Autodesk Inventor part; units mm, degrees
ref_plane "YZ Plane" through (0, 0, 0) normal (1, 0, 0) x (0, 1, 0)
ref_plane "XZ Plane" through (0, 0, 0) normal (0, 1, 0) x (-1, 0, 0)
ref_plane "XY Plane" through (0, 0, 0) normal (0, 0, 1) x (1, 0, 0)
sketch "Sketch1" plane through (0, 0, 0) normal (0, 0, 1) x (1, 0, 0)
  circle A0 centre (0, 0) radius 83.5
  circle A1 centre (0, 0) radius 140
  dimension "d22" = 167
  dimension "d23" = 280
extrude "Plate1" add sketch "Sketch1" along normal blind 4
sketch "Sketch5" plane through (0, 0, 4) normal (0, 0, 1) x (1, 0, 0)
  circle A0 centre (84.8528, 84.8528) radius 9
  circle A1 centre (0, 0) radius 120 construction
  line L0 (84.8528, 84.8528) -> (0, 0) construction
  line L1 (0, 0) -> (0, 120) construction
  dimension "d24" = 18
  dimension "d25" = 240
  dimension "d31" = 45
extrude "Cut1" cut sketch "Sketch5" against normal blind 4
pattern_circular "Circular Pattern1" count 8 over 360 about axis through (0, 0, 0) along (0, 0, 1) of "Cut1"
equation "\"d22\" = Flange_Tube_diam"
equation "\"d23\" = Flange_D_outer"
equation "\"d24\" = Flange_d_hole_diam"
equation "\"d25\" = Flange_D1_hole_center"
equation "\"d26\" = Thickness"
equation "\"d2\" = Thickness"
equation "\"BendReliefWidth\" = Thickness"
equation "\"BendReliefDepth\" = 0.5 * Thickness"
equation "\"CornerReliefSize\" = 4 * Thickness"
equation "\"MinimumRemnant\" = 2 * Thickness"
equation "\"TransitionRadius\" = BendRadius"
equation "\"JacobiRadiusSize\" = BendRadius"
equation "\"GapSize\" = Thickness"
equation "\"Flange_D_outer\" = 280"
equation "\"Flange_D1_hole_center\" = 240"
equation "\"Flange_d_hole_diam\" = 18"
properties part number "drain flange" material "Stainless Steel"
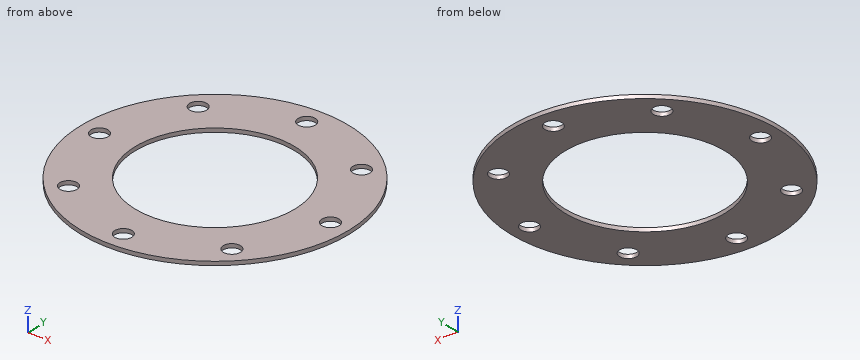
Check sheet for the modelled part. Datum: model origin and axes. Units: mm. Round coordinates to 2 decimals unless told otherwise and drop trailing zeros. Order: outer loops, then holes, each group sorted by start corner. A loop starts at its lowest first (then second) coordinate and runs counter-clockwise, first axis right, second up.
1) Section check A-A (y = 0). Record the boundary of the cut face in (x, z).
2) Section check D-D (z = 1.7). Give the number of separate pieces and of enclosed holes in the cut face, and give its area (3 significant figures).
3) Section check C-C (x = 38.5). Record the boundary of the cut face in (y, z).
4) Go/stop test with flat-tipped pins: pin 1 Ø11 at (x, y) = (-84.85, -84.85) entering from -Z; pin 2 Ø1.5 at (y, z) = (111.5, 2) entering from -X; pin 3 Ø1 at (y, z) = (-86, 1) entering from +X. Record where each tip stops, or that it passes through.
5) Scan lines: line 1 (Y direction, x = 0, z = 1.8); line 2 (X direction, y = -2, z = 0.3); line 3 (X direction, y = 51, z = 2.85). Record each from-to range of solid material in increasing order.
Result:
1. outline: (-140, 0) - (-129, 0) - (-129, 4) - (-140, 4) - close; (-111, 0) - (-83.5, 0) - (-83.5, 4) - (-111, 4) - close; (83.5, 0) - (111, 0) - (111, 4) - (83.5, 4) - close; (129, 0) - (140, 0) - (140, 4) - (129, 4) - close
2. separate pieces: 1
2. enclosed holes: 9
2. area: 37,600 mm2
3. outline: (-134.6, 0) - (-74.09, 0) - (-74.09, 4) - (-134.6, 4) - close; (74.09, 0) - (134.6, 0) - (134.6, 4) - (74.09, 4) - close
4. pin 1: passes through
4. pin 2: stops at x = -85.64
4. pin 3: stops at x = 110.86
5. line 1: y = -140 to -129, -111 to -83.5, 83.5 to 111, 129 to 140
5. line 2: x = -139.99 to -128.77, -111.23 to -83.48, 83.48 to 111.23, 128.77 to 139.99
5. line 3: x = -130.38 to -66.12, 66.12 to 130.38
